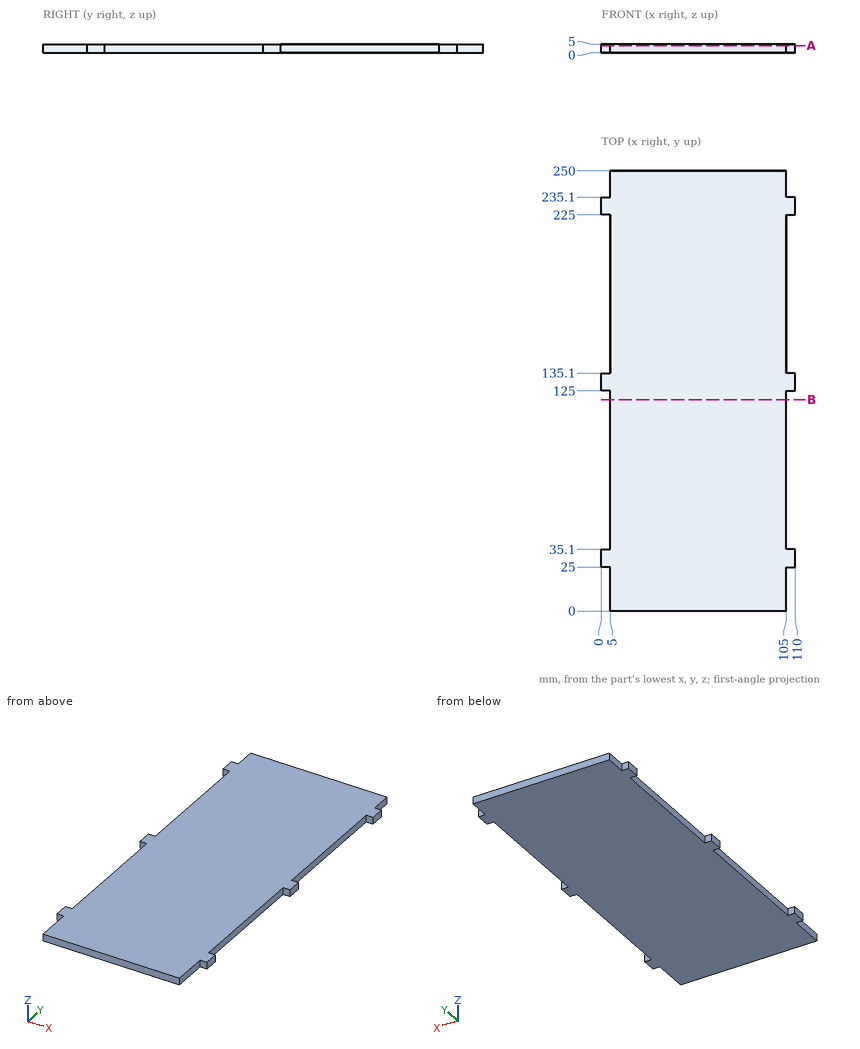
Verification items for this drawing (mm, ordinates from the low corner). Give positions to 0.01 mm unless a question says otherwise; leave off trailing zeros. Write each loop counter-clockwise with the first axis right and the second up, starting at its lowest first coordinate (ties: lowest second). Pieces come first, ordered by that corner, then holes. Notation, with made-up numbers: (2.5, 48.5) -> (33.5, 48.5) arc R31 cw to (33.5, 73.5) -> close; hole circle Ø1 at (44, 62.25). An arc over 180 degrees is marked (long way). Use CSV: the item, a comma, the result in double quotes. Start each with the question number.
Q1. Depth check by flat-ended pin: P1, Ø1.5, axis at x = 108, z = 2, coming from the -Y side; P2, Ø1.5, axis at y = 83, z = 2, coming from the -X side; P3, Ø5, axis at x = 52.5, y = 87, coming from the -Z side; P4, Ø2.5, axis at y = 168.5, z = 2.5, coming from the +X side. Enter the tip coordinate at first touch or a pass-through.
Q2. Cross-section at B-B on y = 120. Enter the section's corners in (x, z).
Q3. Cross-section at A-A on z = 4.05. Enter the section's corners in (x, y).
Q4. Scan line: line 1 along X through (y, z) = (17, 1.1). Record every from-to range of solid material in increasing order.
Working result:
1,P1,"stops at y = 25"
1,P2,"stops at x = 5"
1,P3,"stops at z = 0"
1,P4,"stops at x = 105"
2,outline,"(5, 0) -> (105, 0) -> (105, 5) -> (5, 5) -> close"
3,outline,"(0, 25) -> (5, 25) -> (5, 0) -> (105, 0) -> (105, 25) -> (110, 25) -> (110, 35.1) -> (105, 35.1) -> (105, 125) -> (110, 125) -> (110, 135.1) -> (105, 135.1) -> (105, 225) -> (110, 225) -> (110, 235.1) -> (105, 235.1) -> (105, 250) -> (5, 250) -> (5, 235.1) -> (0, 235.1) -> (0, 225) -> (5, 225) -> (5, 135.1) -> (0, 135.1) -> (0, 125) -> (5, 125) -> (5, 35.1) -> (0, 35.1) -> close"
4,line 1,"x = 5 to 105"
